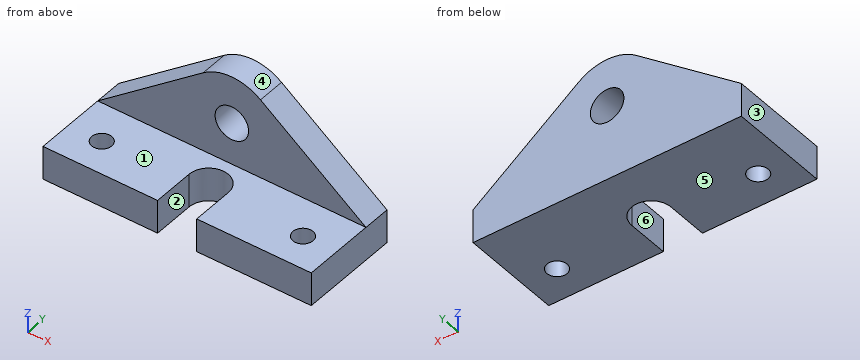
from build123d import *

# Parameters (mm, degrees)
F1_DEPTH = 12
F2_R     = 3.6
F3_DEPTH = 12.001
F4_W     = 96
F4_H     = 10
F5_DEPTH = 32
F6_R     = 6
F7_DEPTH = 10.001
F9_DEPTH = 25


with BuildPart() as f1:
    # F0 (on Top) → F1 (new body)
    with BuildSketch(Plane.XY):
        with BuildLine():
            Line((7, -18), (48, -18))
            Line((48, -18), (48, 18))
            Line((48, 18), (-48, 18))
            Line((-48, 18), (-48, -18))
            Line((-48, -18), (-7, -18))
            Line((-7, -18), (-7, -3))
            ThreePointArc((-7, -3), (0, 4), (7, -3))
            Line((7, -3), (7, -18))
        make_face()
    extrude(amount=F1_DEPTH)

    # F2 (on face) → F3 (cut, through all)
    with BuildSketch(Plane.XY.offset(12)):
        with Locations((36, -6)):
            Circle(F2_R)
        with Locations((-36, -6)):
            Circle(F2_R)
    extrude(amount=-F3_DEPTH, mode=Mode.SUBTRACT)

    # F4 (on face) → F5 (join)
    with BuildSketch(Plane.XY.offset(12)):
        with Locations((0, 13)):
            Rectangle(F4_W, F4_H)
    extrude(amount=F5_DEPTH)

    # F6 (on face) → F7 (cut, through all)
    with BuildSketch(Plane.XZ.offset(-8)):
        with Locations((0, 27)):
            Circle(F6_R)
    extrude(amount=-F7_DEPTH, mode=Mode.SUBTRACT)

    # F8 (on face) → F9 (cut)
    with BuildSketch(Plane.XZ.offset(-8)):
        with BuildLine():
            ThreePointArc((-10.257336, 40.556809), (0, 44), (10.257336, 40.556809))
            Line((10.257336, 40.556809), (48, 12))
            Line((48, 12), (48, 44.921719))
            Line((48, 44.921719), (-48, 44.921719))
            Line((-48, 44.921719), (-48, 12))
            Line((-48, 12), (-10.257336, 40.556809))
        make_face()
    extrude(amount=-F9_DEPTH, mode=Mode.SUBTRACT)


solid = f1.part
Work out the finished part from the listing and answer in its coordinate system (mm). Face numbers are marked on the shaded views. A direction names the side the tool comes from. Coordinates: 2 decimals unless noted, no trailing zeros. Order: outer loops, then holes, each group sorted by start corner. A loop starts at its lowest first (then second) coordinate and runs counter-clockwise, first axis right, second up. Notation, with made-up numbers: (43.5, 2.5) - (49.5, 2.5) arc R26 cw to (49.5, 34.5) - close; hole circle Ø6 at (79, 9.5). An arc over 180 degrees is marked (long way). Put each result on its own line as item: value. Start each with the question number.
1) Flat-ended cylindrical pins translate along their axes: pin 1 (12 mm diameter, centred on x = -28.5, y = 12, fed in from +Z); pin 2 (1 mm diameter, centred on x = 30.5, y = 2, fed in from +Z); pin 3 (4 mm diameter, centred on y = 11, z = 38, fed in from +X); pin 4 (6 mm diameter, centred on y = 4.5, z = 23, fed in from +X). Find the tip coordinate at first contact, or state that the pin passes through.
2) For a pull along X with two mould halves and no side action, classify the marked faces 4, 5 and 6 as released by +X, released by -X, zero draft, split by the parting line, or undercut.
3) Find section D-D (y = -6). Give the vertices of the cut face in (x, z).
4) Find section C-C (z = 7). Give the vertices of the cut face in (x, y), plus the area to 3 significant figures.
5) Find section B-B (x = 0). Give the vertices of the cut face in (y, z).
6) Find the intervals of material crossed by line 1 (Y direction, x = 36, z = 8.5); line 2 (Z direction, x = 0, y = 15); line 3 (Y direction, x = -8.5, z = 28), in increasing order. Write a range as from..to.
7) Find section A-A (y = -14.5). Give the vertices of the cut face in (x, z).
8) For the marked faces 1, 2 and 3, determine the directions among +Z, -Z, +X, -X, +Y, -Y from which every point of the face is accessible in a straight line to the end or side of a thin tool.
Results list:
1. pin 1: stops at z = 31.29
1. pin 2: stops at z = 12
1. pin 3: stops at x = 16.28
1. pin 4: passes through
2. face 4: split by the parting line
2. face 5: zero draft
2. face 6: undercut
3. outline: (-48, 0) - (-39.6, 0) - (-39.6, 12) - (-48, 12) - close; (-32.4, 0) - (-7, 0) - (-7, 12) - (-32.4, 12) - close; (7, 0) - (32.4, 0) - (32.4, 12) - (7, 12) - close; (39.6, 0) - (48, 0) - (48, 12) - (39.6, 12) - close
4. outline: (-48, -18) - (-7, -18) - (-7, -3) arc R7 cw to (7, -3) - (7, -18) - (48, -18) - (48, 18) - (-48, 18) - close; hole circle Ø7.2 at (-36, -6); hole circle Ø7.2 at (36, -6)
4. area: 3,090 mm^2
5. outline: (4, 0) - (18, 0) - (18, 21) - (8, 21) - (8, 12) - (4, 12) - close; (8, 33) - (18, 33) - (18, 44) - (8, 44) - close
6. line 1: y = -18..-9.6, -2.4..18
6. line 2: z = 0..21, 33..44
6. line 3: y = 8..18
7. outline: (-48, 0) - (-7, 0) - (-7, 12) - (-48, 12) - close; (7, 0) - (48, 0) - (48, 12) - (7, 12) - close
8. face 1: +Z, +X, -X, -Y
8. face 2: +Z, -Z, -Y
8. face 3: +Z, -Z, -X, +Y, -Y
